Geometry check sheet. Reference: drawing and pictorial views, mm from the part's lowest x, y, z. Coordinates: 2 decimals unless noted, no trailing zeros. Loops run counter-clockwise (first coordinate to the right, second up) from the corner with the lowest first, then second, coordinate; pieces in that order, holes last. Notation, with made-up numbers: (11.5, -17.5) - (54.5, -17.5) arc R24 ccw to (54.5, 13.5) - close; hole circle Ø2 at (-30, -1). An arc over 180 degrees is marked (long way). Use a Markdown table: item, result. Add a question column.
1) Go/stop test with flat-tipped pins: P1, Ø1.5, axis at x = 8, z = 6, coming from the -Y side; P2, Ø1.5, axis at x = 50.5, y = 11, coming from the -Z side; P3, Ø10, axis at x = 50.5, y = 18, coming from the +Z side. Record where each tip stops, or that it passes through.
2) Sectioned sample at D-D, the plane y = 27.75. Enter the section's corners in (x, z).
3) Sectioned sample at B-B, the plane z = 9. Enter the section's corners in (x, y), then the cut area to 3 significant figures.
4) Sectioned sample at A-A, the plane y = 18.5. Enter the section's corners in (x, z).
5) Sectioned sample at C-C, the plane x = 20. Enter the section's corners in (y, z), then the cut area to 3 significant figures.
6) Thickness scan on line 1 (X direction, y = 5.5, z = 9); line 2 (Y direction, x = 7.5, z = 8.5); line 3 (Z direction, x = 6.5, y = 26). Record the ranges inside material, lowest first.
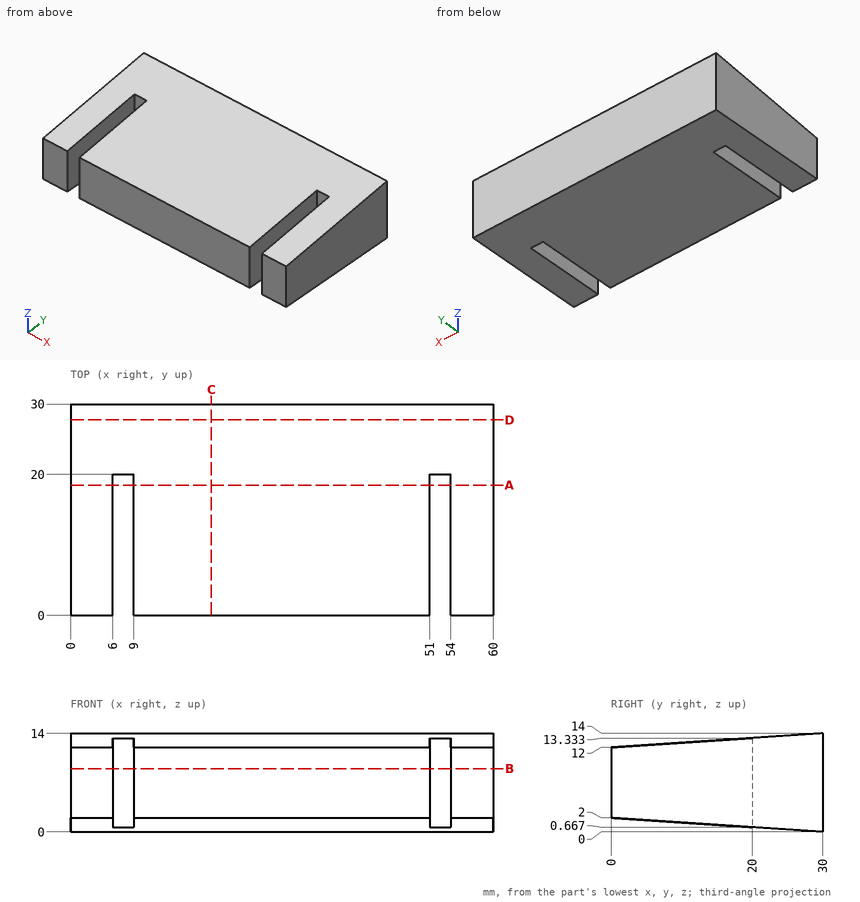
Solved:
| question | item | result |
|---|---|---|
| 1 | P1 | stops at y = 20 |
| 1 | P2 | stops at z = 1.22 |
| 1 | P3 | stops at z = 13.53 |
| 2 | outline | (0, 0.15) - (60, 0.15) - (60, 13.85) - (0, 13.85) - close |
| 3 | outline | (0, 0) - (6, 0) - (6, 20) - (9, 20) - (9, 0) - (51, 0) - (51, 20) - (54, 20) - (54, 0) - (60, 0) - (60, 30) - (0, 30) - close |
| 3 | area | 1,680 mm2 |
| 4 | outline | (0, 0.77) - (6, 0.77) - (6, 13.23) - (0, 13.23) - close; (9, 0.77) - (51, 0.77) - (51, 13.23) - (9, 13.23) - close; (54, 0.77) - (60, 0.77) - (60, 13.23) - (54, 13.23) - close |
| 5 | outline | (0, 2) - (30, 0) - (30, 14) - (0, 12) - close |
| 5 | area | 360 mm2 |
| 6 | line 1 | x = 0 to 6, 9 to 51, 54 to 60 |
| 6 | line 2 | y = 20 to 30 |
| 6 | line 3 | z = 0.27 to 13.73 |
